Autodesk Inventor part; units mm, degrees
ref_plane "YZ Plane" through (0, 0, 0) normal (1, 0, 0) x (0, 1, 0)
ref_plane "XZ Plane" through (0, 0, 0) normal (0, 1, 0) x (-1, 0, 0)
ref_plane "XY Plane" through (0, 0, 0) normal (0, 0, 1) x (1, 0, 0)
sketch "Sketch1" plane through (0, 0, 0) normal (0, 0, 1) x (1, 0, 0)
  line L0 (0, 10) -> (6, 10)
  line L1 (6, 10) -> (6, 4)
  line L2 (6, 4) -> (15, 4)
  line L3 (15, 4) -> (15, 0)
  line L4 (15, 0) -> (0, 0)
  line L5 (0, 0) -> (0, 10)
  dimension "d0" = 4
  dimension "d1" = 10
  dimension "d2" = 15
  dimension "d3" = 6
revolve "Revolution1" add sketch "Sketch1" angle 360 about axis through (0, 0, 0) along (0, 1, 0)
sketch "Sketch2" plane through (0, 10, 0) normal (0, 1, 0) x (1, 0, 0)
  circle A0 centre (0, 0) radius 6
  line L0 (0, 6) -> (0, 15)
  circle A1 centre (0, 0) radius 15
  circle A2 centre (0, 0) radius 6
  circle A3 centre (0, 0) radius 15
  line L1 (0, -6) -> (0, -15)
  point P0 (0, 10.5)
  point P1 (0, -10.5)
  point P2 (0, -10.5)
  point P3 (0, 10.5)
hole "Hole1" at (0, 10, 0) direction (0, -1, 0) diameter 8 end through all
hole "Hole2" at (0, 10, -10.5) at (0, 10, 10.5) direction (0, -1, 0) diameter 4.134 end through all
sketch "Sketch3" plane through (0, 0, 0) normal (1, 0, 0) x (0, 1, 0)
  line L0 (10, 6) -> (10, -6)
  line L1 (4, 6) -> (4, -6)
  line L2 (4, 15) -> (4, -15)
  line L3 (0, 15) -> (0, -15)
  line L4 (10, 0) -> (4, 0)
  line L5 (4, 6) -> (4, -6)
  point P0 (0, 0)
  point P1 (7, 0)
  point P2 (7, 0)
hole "Hole3" at (0, 7, 0) direction (1, 0, 0) diameter 2.459 end through all
sketch "Sketch4" plane through (0, 0, 0) normal (0, 0, 1) x (1, 0, 0)
  line L0 (-15, 4) -> (15, 4)
  line L1 (-15, 0) -> (15, 0)
  line L2 (-4, 10) -> (4, 10)
  line L3 (0, 10) -> (0, 4)
  line L4 (-6, 4) -> (6, 4)
  point P0 (0, 0)
  point P1 (0, 7)
hole "Hole4" at (0, 7, 0) direction (0, 0, -1) diameter 2.459 end through all
properties part number "asbevestiging" material "Aluminum 6061"
Geometry: final body of the model. Coordinates: model frame, mm. A direction names the side the tool comes from. Round coordinates to 2 decimals unless told otherwise and drop trailing zeros. Order: outer loops, then holes, each group sorted by start corner. A loop starts at its lowest first (then second) coordinate and runs counter-clockwise, first axis right, second up. Notation, with made-up numbers: (26, 38) -> (59, 38) arc R26 cw to (59, 70) -> close; hole circle Ø9 at (-26, 49). An arc over 180 degrees is marked (long way). Use one line per item in the form item = value. Start each with the question number.
1. Cut plane D-D (y = 9). Return the cut outline in (x, z).
2. Cut plane B-B (z = 10.5). Return the cut outline in (x, y).
3. Draft query along Z for faces 4 (the face through (-1.201, 4.93, 3.815)), 5 (the face through (-6, 7, 0)), 6 (the face through (-0.2, 4, 6.5)). Return one class per face: pulls with the +Z half, pulls with the -Z half, needs draft (parallel to the pull), parting line crosses it, or undercut.
4. Pin query (flat end, axial travel): pin 1 Ø3 at (x, y) = (0, 7) entering from +Z; pin 2 Ø3.5 at (x, z) = (0, -10.5) entering from -Y; pin 3 Ø2 at (x, y) = (-9.5, 1.5) entering from +Z; pin 4 Ø5 at (x, z) = (0, 10.5) entering from +Y. Return the tip coordinate at first contact, or that it passes through.
5. Cut plane A-A (x = 0). Return the cut outline in (y, z), then the cut area to 3 significant figures.
6. Line query: probe 1 along Z at (x, y) = (0, 2.3); probe 2 along Y at (x, z) = (4.85, 0); probe 3 along Y at (x, z) = (-12.25, 0). Output: solid intervals per line, ascending.
7. Cut plane C-C (y = 7). Return the cut outline in (x, z).
8. Reachability of faces 1 (the face through (-0.091, 1.972, 8.435)), 2 (the face through (4.92, 6.95, -1.23)), 3 (the face through (-0.05, 8.23, -4.92)) from +Z, -Z, +X, -X, +Y, -Y: full face, straight path, thin tool, end or side. Return the list, or none.
Solution:
q1.outline = circle Ø12 at (0, 0); hole circle Ø8 at (0, 0)
q2.outline = (-10.71, 0) -> (-2.07, 0) -> (-2.07, 4) -> (-10.71, 4) -> close; (2.07, 0) -> (10.71, 0) -> (10.71, 4) -> (2.07, 4) -> close
q3.face_4 = undercut
q3.face_5 = parting line crosses it
q3.face_6 = needs draft
q4.pin_1 = 6
q4.pin_2 = through
q4.pin_3 = 12.36
q4.pin_4 = 4
q5.outline = (0, -15) -> (4, -15) -> (4, -12.57) -> (0, -12.57) -> close; (0, -8.43) -> (4, -8.43) -> (4, -6) -> (5.77, -6) -> (5.77, -4) -> (0, -4) -> close; (0, 4) -> (10, 4) -> (10, 6) -> (4, 6) -> (4, 8.43) -> (0, 8.43) -> close; (0, 12.57) -> (4, 12.57) -> (4, 15) -> (0, 15) -> close; (8.23, -6) -> (10, -6) -> (10, -4) -> (8.23, -4) -> close
q5.area = 74.0 mm^2
q6.probe_1 = -15 to -12.57, -8.43 to -4, 4 to 8.43, 12.57 to 15
q6.probe_2 = 0 to 5.77, 8.23 to 10
q6.probe_3 = 0 to 4
q7.outline = (-1.23, -5.87) -> (-1.23, -3.81) arc R4 cw (long way) to (3.81, 1.23) -> (5.87, 1.23) arc R6 ccw (long way) to start; (1.23, -5.87) arc R6 ccw to (5.87, -1.23) -> (3.81, -1.23) arc R4 cw to (1.23, -3.81) -> close
q8.face_1 = +Y, -Y
q8.face_2 = +X
q8.face_3 = -Z
